Input: part model. Units: mm. Frame: model coordinates. A direction names the side the tool comes from. Coordinates: 2 decimals unless noted, no trailing zeros. Write each loop counter-clockwise with the first axis right and the second up, starting at its lowest first coordinate (ties: lowest second). Pieces come first, ordered by that corner, then holes. Notation, with made-up numbers: M -21.5,44.5 L -17.5,44.5 A14 ccw -17.5,71.5 Z; hole C 43.25,29.5 d2. An arc over 180 degrees is marked long. Use CSV: the item, a comma, the result in double quotes.
```python
from build123d import *

# Parameters (mm, degrees)
EXTRUDE_1_DEPTH     = 10
SKETCH_4_W          = 28
SKETCH_4_H          = 100
EXTRUDE_2_DEPTH     = 20
SKETCH_5_R          = 5
CUT_EXTRUDE_2_DEPTH = 30
SKETCH_9_R          = 2.4
CUT_EXTRUDE_4_DEPTH = 10
SKETCH_10_R         = 6
CUT_EXTRUDE_5_DEPTH = 10


with BuildPart() as part:
    # 草图1 → 凸台-拉伸1 (new body)
    with BuildSketch(Plane(origin=(0, 0, 0), x_dir=(1, 0, 0), z_dir=(0, 1, 0))):
        Polygon((0, -50), (125, -50), (125, 50), (-125, 50), (-125, -50), align=None)
    extrude(amount=EXTRUDE_1_DEPTH)

    # 草图4 → 凸台-拉伸2 (add)
    with BuildSketch(Plane.XZ):
        with Locations((-111, 0)):
            Rectangle(SKETCH_4_W, SKETCH_4_H)
    extrude_2 = extrude(amount=EXTRUDE_2_DEPTH)

    # 镜向1: 凸台-拉伸2 across plane
    add(extrude_2.mirror(Plane(origin=(0, 0, 0), x_dir=(0, 0, 1), z_dir=(1, 0, 0))))

    # 草图5 → 切除-拉伸2 (cut)
    with BuildSketch(Plane(origin=(125, 0, 0), x_dir=(0, 0, -1), z_dir=(1, 0, 0))):
        with Locations((0, -10)):
            Circle(SKETCH_5_R)
        with Locations((-35, -10)):
            Circle(SKETCH_5_R)
        with Locations((35, -10)):
            Circle(SKETCH_5_R)
    cut_extrude_2 = extrude(amount=-CUT_EXTRUDE_2_DEPTH, mode=Mode.SUBTRACT)

    # 镜向2: 切除-拉伸2 across plane
    add(cut_extrude_2.mirror(Plane(origin=(0, 0, 0), x_dir=(0, 0, 1), z_dir=(1, 0, 0))), mode=Mode.SUBTRACT)

    # 草图9 → 切除-拉伸4 (cut)
    with BuildSketch(Plane(origin=(0, 10, 0), x_dir=(1, 0, 0), z_dir=(0, 1, 0))):
        with Locations(Location((0, 24, 0), (0, 0, 270))):
            Circle(SKETCH_9_R)
        with Locations(Location((20.784609691, -12, 0), (0, 0, 270))):
            Circle(SKETCH_9_R)
        with Locations(Location((-20.784609691, -12, 0), (0, 0, 270))):
            Circle(SKETCH_9_R)
    extrude(amount=-CUT_EXTRUDE_4_DEPTH, mode=Mode.SUBTRACT)

    # 草图10 → 切除-拉伸5 (cut)
    with BuildSketch(Plane(origin=(0, 10, 0), x_dir=(1, 0, 0), z_dir=(0, 1, 0))):
        with Locations(Location((0, 0, 0), (0, 0, 270))):
            Circle(SKETCH_10_R)
    extrude(amount=-CUT_EXTRUDE_5_DEPTH, mode=Mode.SUBTRACT)


solid = part.part
```
1. Contact query for flat-ended pins moving along their axis: pin 1 Ø6 at (y, z) = (-10, 35) entering from -X; pin 2 Ø8 at (x, z) = (28.5, 30) entering from -Y. Output: stop coordinate, or through.
Resolved:
pin 1,"passes through"
pin 2,"stops at y = 0"
2. Section D-D (z = 35). Return loops of the section in (x, y).
Resolved:
outline,"M -125,-20 L -97,-20 L -97,-15 L -125,-15 Z; M -125,-5 L -97,-5 L -97,0 L 97,0 L 97,-5 L 125,-5 L 125,10 L -125,10 Z; M 97,-20 L 125,-20 L 125,-15 L 97,-15 Z"
3. Section C-C (z = 0). Return loops of the section in (x, y).
Resolved:
outline,"M -125,-20 L -97,-20 L -97,-15 L -125,-15 Z; M -125,-5 L -97,-5 L -97,0 L -6,0 L -6,10 L -125,10 Z; M 6,0 L 97,0 L 97,-5 L 125,-5 L 125,10 L 6,10 Z; M 97,-20 L 125,-20 L 125,-15 L 97,-15 Z"
4. Access query for faces 1 (the flat face through (97, -3, -1)), 2 (the flat face through (-111, -20, 1)). Directions: +Z, -Z, +X, -X, +Y, -Y. A direction counts if a zero-diameter tool reaches every point of the face in a straight line with its end or side. Return the directions, or none.
Resolved:
face 1,"+Z, -Z, -Y"
face 2,"+Z, -Z, +X, -X, -Y"
5. Section A-A (x = 0). Return loops of the section in (y, z).
Resolved:
outline,"M 0,-50 L 10,-50 L 10,-26.4 L 0,-26.4 Z; M 0,-21.6 L 10,-21.6 L 10,-6 L 0,-6 Z; M 0,6 L 10,6 L 10,50 L 0,50 Z"
6. Section B-B (z = -24). Return loops of the section in (x, y), then the cut area to 3 significant figures.
Resolved:
outline,"M -125,-20 L -97,-20 L -97,0 L -2.4,0 L -2.4,10 L -125,10 Z; M 2.4,0 L 97,0 L 97,-20 L 125,-20 L 125,10 L 2.4,10 Z"
area,"3,570 mm^2"
7. Mould query, pull axis Z, two halves, no side actions, for faces 3 (the flat face through (-97, -3, -1)), 4 (the cylindrical face through (111, -10, -30)), 5 (the flat face through (2, 2, 50)). Classes: pulls with the +Z half, pulls with the -Z half, needs draft (parallel to the pull), parting line crosses it, or undercut.
Resolved:
face 3,"needs draft"
face 4,"undercut"
face 5,"pulls with the +Z half"
8. Material intervals for line 1 (Z direction, x = -117.25, y = -10); line 2 (X direction, y = 6.25, z = 12); line 3 (X direction, y = -11.5, z = -43.5), sorted ascending. Write a range as [from, to].
Resolved:
line 1,"z = [-50, -40], [-30, -5], [5, 30], [40, 50]"
line 2,"x = [-125, -23.18], [-18.38, 18.38], [23.18, 125]"
line 3,"x = [-125, -97], [97, 125]"
